Read the model definition and answer for the solid it produces. Units are mm, in the model's axes. Face numbers are marked on the shaded views. A direction names the side the tool comes from. Coordinates: 2 decimals unless noted, no trailing zeros. Loops run counter-clockwise (first coordinate to the right, second up) from the corner with the lowest first, then second, coordinate; pieces in that order, holes last.
Q1. Flat-ended cylindrical pins translate along their axes: P1, Ø5, axis at y = 10.5, z = -4, coming from the +X side; P2, Ø1.5, axis at x = -19.5, y = 7.5, coming from the +Z side; P3, Ø1.6, axis at x = -29.5, y = 13, coming from the -Z side. Find the tip coordinate at first contact, or state that the pin passes through.
Q2. Section B-B (z = -6.5) is taken. Give the vertices of the cut face in (x, y), then the cut area to 3 significant figures.
Q3. Section C-C (y = 14.5) is taken. Give the vertices of the cut face in (x, z).
Q4. Section A-A (x = -34) is taken. Give the vertices of the cut face in (y, z).
Q5. Section D-D (x = -14.5) is taken. Give the vertices of the cut face in (y, z).
Q6. The mould has two halves that part along Y. Classify the marked faces 4, 5 and 6: pulls with the +Y half, pulls with the -Y half, needs draft (parallel to the pull), parting line crosses it, or undercut.
Q7. Straight lines are drawn through the part: line 1 (X direction, y = 17.5, z = -2.75); line 2 (X direction, y = 9.75, z = 9); line 3 (Y direction, x = 9.5, z = 0.5). For each, find the intervals that lie inside material, in ascending order.
Q8. Which of the six approach directions +Z, -Z, +X, -X, +Y, -Y give full straight-line access (tool end or side, diameter ignored) to the marked faces 1, 2 and 3?
from build123d import *

# Parameters (mm, degrees)
SKETCH1_W           = 76
SKETCH1_H           = 21
BOSS_EXTRUDE1_DEPTH = 4
SKETCH2_W           = 76
SKETCH2_H           = 3.8
BOSS_EXTRUDE2_DEPTH = 26
SKETCH3_W           = 62
SKETCH3_H           = 22
BOSS_EXTRUDE3_DEPTH = 15.7
CHAMFER2_SIZE       = 2
SKETCH4_W           = 55.8
SKETCH4_H           = 8.6
CUT_EXTRUDE1_DEPTH  = 0.6
CUT_EXTRUDE2_DEPTH  = 46.14698218
SKETCH6_W           = 8
SKETCH6_H           = 4
CUT_EXTRUDE3_DEPTH  = 19.7
SKETCH7_W           = 58
SKETCH7_H           = 15.4
CUT_EXTRUDE4_DEPTH  = 13.7
CUT_EXTRUDE5_DEPTH  = 13.7
LPATTERN1_COUNT     = 3
LPATTERN1_PITCH     = 25.8
BOSS_EXTRUDE4_REACH = 52.606
SKETCH9_W           = 1.9
SKETCH9_H           = 15.4
CUT_EXTRUDE6_REACH  = 53.418
CUT_EXTRUDE7_REACH  = 76.48
SKETCH12_W          = 1.2
SKETCH12_H          = 3.8
CUT_EXTRUDE8_DEPTH  = 11.9


with BuildPart() as part:
    # Sketch1 → Boss-Extrude1 (new body)
    with BuildSketch(Plane(origin=(0, 0, 0), x_dir=(1, 0, 0), z_dir=(0, 1, 0))):
        Rectangle(SKETCH1_W, SKETCH1_H)
    extrude(amount=BOSS_EXTRUDE1_DEPTH)

    # Sketch2 → Boss-Extrude2 (add)
    with BuildSketch(Plane(origin=(0, 0, 0), x_dir=(1, 0, 0), z_dir=(0, 1, 0))):
        with Locations((0, -8.6)):
            Rectangle(SKETCH2_W, SKETCH2_H)
    extrude(amount=BOSS_EXTRUDE2_DEPTH)

    # Sketch3 → Boss-Extrude3 (add)
    with BuildSketch(Plane(origin=(0, 0, 10.5), x_dir=(-1, 0, 0), z_dir=(0, 0, -1))):
        with Locations((0, 15)):
            Rectangle(SKETCH3_W, SKETCH3_H)
    extrude(amount=BOSS_EXTRUDE3_DEPTH)

    # Chamfer2
    chamfer2_edges = [part.edges().sort_by_distance(p)[0] for p in [
        (-38, 2, -10.5),
        (38, 2, -10.5),
    ]]
    chamfer(chamfer2_edges, length=CHAMFER2_SIZE)

    # Sketch4 → Cut-Extrude1 (cut)
    with BuildSketch(Plane(origin=(0, 26, 0), x_dir=(1, 0, 0), z_dir=(0, 1, 0))):
        with Locations((0, -1.9)):
            Rectangle(SKETCH4_W, SKETCH4_H)
    extrude(amount=-CUT_EXTRUDE1_DEPTH, mode=Mode.SUBTRACT)

    # Sketch5 → Cut-Extrude2 (cut, through all)
    with BuildSketch(Plane(origin=(0, 4, 0), x_dir=(1, 0, 0), z_dir=(0, 1, 0))):
        with BuildLine():
            Line((-32, 2.7), (-32, -3.3))
            ThreePointArc((-32, -3.3), (-34, -5.3), (-36, -3.3))
            Line((-36, -3.3), (-36, 2.7))
            ThreePointArc((-36, 2.7), (-34, 4.7), (-32, 2.7))
        make_face()
        with BuildLine():
            Line((32, 2.7), (32, -3.3))
            ThreePointArc((32, -3.3), (34, -5.3), (36, -3.3))
            Line((36, -3.3), (36, 2.7))
            ThreePointArc((36, 2.7), (34, 4.7), (32, 2.7))
        make_face()
    extrude(amount=-CUT_EXTRUDE2_DEPTH, mode=Mode.SUBTRACT)

    # Sketch6 → Cut-Extrude3 (cut)
    with BuildSketch(Plane(origin=(0, 0, -10.5), x_dir=(-1, 0, 0), z_dir=(0, 0, -1))):
        with Locations((-12.75, 3.1)):
            Rectangle(SKETCH6_W, SKETCH6_H)
        with Locations((12.75, 3.1)):
            Rectangle(SKETCH6_W, SKETCH6_H)
    extrude(amount=-CUT_EXTRUDE3_DEPTH, mode=Mode.SUBTRACT)

    # Sketch7 → Cut-Extrude4 (cut)
    with BuildSketch(Plane.XY.offset(10.5)):
        with Locations((0, 13)):
            Rectangle(SKETCH7_W, SKETCH7_H)
    extrude(amount=-CUT_EXTRUDE4_DEPTH, mode=Mode.SUBTRACT)

    # Sketch8 → Cut-Extrude5 (cut)
    with BuildSketch(Plane.XY.offset(10.5)):
        with BuildLine():
            Line((-29, 23), (-29, 3))
            ThreePointArc((-29, 3), (-25.8, 2.15), (-22.6, 3))
            Line((-22.6, 3), (-22.6, 23))
            ThreePointArc((-22.6, 23), (-25.8, 23.85), (-29, 23))
        make_face()
    cut_extrude5 = extrude(amount=-CUT_EXTRUDE5_DEPTH, mode=Mode.SUBTRACT)

    # LPattern1: Cut-Extrude5 ×3
    with Locations(*[(i * LPATTERN1_PITCH, 0, 0) for i in range(1, LPATTERN1_COUNT)]):
        add(cut_extrude5, mode=Mode.SUBTRACT)

    # Sketch9 → Boss-Extrude4 (add, up to next)
    with BuildSketch(Plane.XY.offset(10.5), mode=Mode.PRIVATE) as boss_extrude4_sk1:
        with Locations((-4.15, 13)):
            Rectangle(SKETCH9_W, SKETCH9_H)
    boss_extrude4_tool1 = extrude(boss_extrude4_sk1.sketch, amount=-BOSS_EXTRUDE4_REACH, mode=Mode.PRIVATE) - part.part
    # Sketch9 → Boss-Extrude4 (add, up to next)
    with BuildSketch(Plane.XY.offset(10.5), mode=Mode.PRIVATE) as boss_extrude4_sk2:
        with Locations((4.15, 13)):
            Rectangle(SKETCH9_W, SKETCH9_H)
    boss_extrude4_tool2 = extrude(boss_extrude4_sk2.sketch, amount=-BOSS_EXTRUDE4_REACH, mode=Mode.PRIVATE) - part.part
    add(boss_extrude4_tool1.solids().sort_by_distance((-4.15, 13, 10.5))[0])
    add(boss_extrude4_tool2.solids().sort_by_distance((4.15, 13, 10.5))[0])

    # Cut-Extrude6: up to this face of the body (flat: up to its plane)
    cut_extrude6_end = Plane(part.part.faces().sort_by_distance((5.1, 13, 3.65))[0])
    # Sketch10 → Cut-Extrude6 (cut, up to the picked face)
    with BuildSketch(Plane.ZY.offset(5.1), mode=Mode.PRIVATE) as cut_extrude6_sk1:
        with BuildLine():
            Line((10.5, 15.25), (1.75, 15.25))
            ThreePointArc((1.75, 15.25), (-0.5, 13), (1.75, 10.75))
            Line((1.75, 10.75), (10.5, 10.75))
            Line((10.5, 10.75), (10.5, 15.25))
        make_face()
    cut_extrude6_tool1 = split(extrude(cut_extrude6_sk1.sketch, amount=-CUT_EXTRUDE6_REACH, mode=Mode.PRIVATE), bisect_by=cut_extrude6_end, keep=Keep.BOTH, mode=Mode.PRIVATE)
    add(cut_extrude6_tool1.solids().sort_by(Axis((-5.1, 13, 5.229437), (1, 0, 0)))[0], mode=Mode.SUBTRACT)

    # Sketch11 → Cut-Extrude7 (cut, up to next)
    with BuildSketch(Plane.ZY.offset(31), mode=Mode.PRIVATE) as cut_extrude7_sk1:
        Polygon((1.5, 17.5), (-2.5, 15.190598923), (-2.5, 10.57179677), (1.5, 8.262395693), (5.5, 10.57179677), (5.5, 15.190598923), align=None)
    cut_extrude7_tool1 = extrude(cut_extrude7_sk1.sketch, amount=-CUT_EXTRUDE7_REACH, mode=Mode.PRIVATE) & part.part
    cut_extrude7 = cut_extrude7_tool1.solids().sort_by_distance((-31, 12.881198, 1.5))[0]
    add(cut_extrude7, mode=Mode.SUBTRACT)

    # Mirror1: Cut-Extrude7 across plane
    add(cut_extrude7.mirror(Plane(origin=(0, 0, 0), x_dir=(0, 0, 1), z_dir=(1, 0, 0))), mode=Mode.SUBTRACT)

    # Sketch12 → Cut-Extrude8 (cut)
    with BuildSketch(Plane(origin=(0, 0, -5.2), x_dir=(-1, 0, 0), z_dir=(0, 0, -1))):
        with Locations((-30.4, 5.9)):
            Rectangle(SKETCH12_W, SKETCH12_H)
        with Locations((30.4, 5.9)):
            Rectangle(SKETCH12_W, SKETCH12_H)
    extrude(amount=-CUT_EXTRUDE8_DEPTH, mode=Mode.SUBTRACT)


solid = part.part
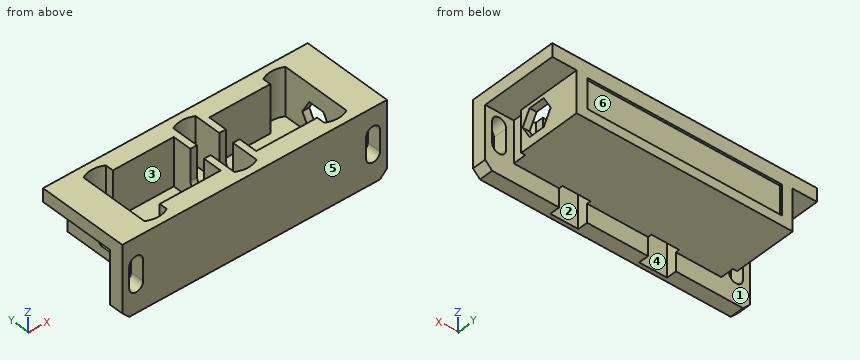
Numbers:
1. P1: stops at x = 31
1. P2: stops at z = -3.2
1. P3: stops at z = -5.2
2. outline: (-38, 0) - (38, 0) - (38, 4) - (16.75, 4) - (16.75, 1.1) - (8.75, 1.1) - (8.75, 4) - (-8.75, 4) - (-8.75, 1.1) - (-16.75, 1.1) - (-16.75, 4) - (-38, 4) - close
2. area: 258 mm2
3. outline: (-38, 6.7) - (-31, 6.7) - (-31, 5.5) - (-29, 5.5) - (-29, 10.5) - (-38, 10.5) - close; (-31, -5.2) - (31, -5.2) - (31, -2.5) - (29, -2.5) - (29, -3.2) - (5.1, -3.2) - (5.1, 0.07) - (3.2, 0.07) - (3.2, -3.2) - (-3.2, -3.2) - (-3.2, 0.07) - (-5.1, 0.07) - (-5.1, -3.2) - (-29, -3.2) - (-29, -2.5) - (-31, -2.5) - close; (29, 5.5) - (31, 5.5) - (31, 6.7) - (38, 6.7) - (38, 10.5) - (29, 10.5) - close
4. outline: (0, -10.5) - (4, -10.5) - (4, -4.7) - (0, -4.7) - close; (0, 5.3) - (4, 5.3) - (4, 6.7) - (26, 6.7) - (26, 10.5) - (0, 10.5) - close
5. outline: (0, -10.5) - (1.1, -10.5) - (1.1, 9.2) - (5.1, 9.2) - (5.1, -5.2) - (26, -5.2) - (26, -2.4) - (25.4, -2.4) - (25.4, 6.2) - (26, 6.2) - (26, 10.5) - (20.7, 10.5) - (20.7, -3.2) - (5.3, -3.2) - (5.3, 10.5) - (0, 10.5) - close
6. face 4: undercut
6. face 5: pulls with the -Y half
6. face 6: pulls with the +Y half
7. line 1: x = -31 to -29, -5.1 to -3.2, 3.2 to 5.1, 29 to 31
7. line 2: x = -38 to -29, -5.1 to -3.2, 3.2 to 5.1, 29 to 38
7. line 3: y = 0 to 1.1, 5.1 to 5.3, 20.7 to 25.4
8. face 1: -Z, -X
8. face 2: -Z
8. face 3: +Z
